```python
from build123d import *

# Parameters (mm, degrees)
F0_W      = 79.8
F0_H      = 79.8
F1_DEPTH  = 15
F2_W      = 74
F2_H      = 74
F3_DEPTH  = 13
F4_W      = 73.8
F4_H      = 73.8
F4_W_2    = 69.8
F4_H_2    = 69.8
F5_DEPTH  = 2
F7_DEPTH  = 2
F8_R      = 2
F9_R      = 4
F10_R     = 0.99999
F12_DEPTH = 79.801
F13_R     = 5
F14_R     = 4
F15_R     = 1


# Not quite as in the source:
# - a fillet or chamfer is up to 0.001 mm smaller than in the source, because OpenCascade refuses the exact size


with BuildPart() as f1:
    # F0 (on Top) → F1 (new body)
    with BuildSketch(Plane.XY):
        Rectangle(F0_W, F0_H)
    extrude(amount=F1_DEPTH)

    # F2 (on face) → F3 (cut)
    with BuildSketch(Plane.XY.offset(15)):
        Rectangle(F2_W, F2_H)
    extrude(amount=-F3_DEPTH, mode=Mode.SUBTRACT)

    # F4 (on face) → F5 (join)
    with BuildSketch(Plane(origin=(0, 0, 0), x_dir=(1, 0, 0), z_dir=(0, 0, -1))):
        Rectangle(F4_W, F4_H)
        Rectangle(F4_W_2, F4_H_2, mode=Mode.SUBTRACT)
    extrude(amount=F5_DEPTH)

    # F6 (on face) → F7 (cut, through all)
    with BuildSketch(Plane(origin=(0, 0, -2), x_dir=(1, 0, 0), z_dir=(0, 0, -1))):
        Polygon((36.9, -21.9), (36.9, 21.9), (21.9, 21.9), (21.9, 36.9), (-21.9, 36.9), (-21.9, 21.9), (-36.9, 21.9), (-36.9, -21.9), (-21.9, -21.9), (-21.9, -36.9), (21.9, -36.9), (21.9, -21.9), align=None)
    extrude(amount=-F7_DEPTH, mode=Mode.SUBTRACT)

    # F8
    f8_edges = [f1.edges().sort_by_distance(p)[0] for p in [
        (-34.9, 34.9, -1),
        (-34.9, -34.9, -1),
        (34.9, -34.9, -1),
        (34.9, 34.9, -1),
    ]]
    fillet(f8_edges, radius=F8_R)

    # F9
    f9_edges = [f1.edges().sort_by_distance(p)[0] for p in [
        (-36.9, 36.9, -1),
        (36.9, 36.9, -1),
        (36.9, -36.9, -1),
        (-36.9, -36.9, -1),
    ]]
    fillet(f9_edges, radius=F9_R)

    # F10 (radius 1 in the source; OpenCascade refuses exactly that, so slightly less here)
    f10_edges = [f1.edges().sort_by_distance(p)[0] for p in [
        (21.9, -35.9, -2),
        (21.9, -35.9, 0),
        (35.9, -21.9, -2),
        (35.9, -21.9, 0),
        (-35.9, -21.9, -2),
        (-35.9, -21.9, 0),
        (-21.9, -35.9, -2),
        (-21.9, -35.9, 0),
        (-35.9, 21.9, -2),
        (-35.9, 21.9, 0),
        (-21.9, 35.9, -2),
        (-21.9, 35.9, 0),
        (21.9, 35.9, -2),
        (21.9, 35.9, 0),
        (35.9, 21.9, -2),
        (35.9, 21.9, 0),
    ]]
    fillet(f10_edges, radius=F10_R)

    # F11 (on face) → F12 (cut, through all)
    with BuildSketch(Plane.XZ.offset(39.9)):
        Polygon((20, 30), (-20, 30), (-12.2222222222, 2), (12.2222222222, 2), align=None)
    extrude(amount=-F12_DEPTH, mode=Mode.SUBTRACT)

    # F13
    f13_edges = [f1.edges().sort_by_distance(p)[0] for p in [
        (-15.833333, 38.45, 15),
        (-15.833333, -38.45, 15),
        (15.833333, -38.45, 15),
        (15.833333, 38.45, 15),
        (-12.222222, 38.45, 2),
        (-12.222222, -38.45, 2),
        (12.222222, -38.45, 2),
        (12.222222, 38.45, 2),
    ]]
    fillet(f13_edges, radius=F13_R)

    # F14
    f14_edges = [f1.edges().sort_by_distance(p)[0] for p in [
        (39.9, -39.9, 7.5),
        (39.9, 39.9, 7.5),
        (-39.9, -39.9, 7.5),
        (-39.9, 39.9, 7.5),
    ]]
    fillet(f14_edges, radius=F14_R)

    # F15
    f15_edges = [f1.edges().sort_by_distance(p)[0] for p in [
        (37, 37, 8.5),
        (-37, 37, 8.5),
        (-37, -37, 8.5),
        (37, -37, 8.5),
    ]]
    fillet(f15_edges, radius=F15_R)


solid = f1.part
```
Work out the finished part from the listing and answer in its coordinate system (mm). A direction names the side the tool comes from. Give positions to 0.01 mm unless a question says otherwise; leave off trailing zeros. Order: outer loops, then holes, each group sorted by start corner. A loop starts at its lowest first (then second) coordinate and runs counter-clockwise, first axis right, second up. Notation, with made-up numbers: (14.25, -3) - (18.25, -3) arc R15 ccw to (18.25, 18) - close; hole circle Ø11 at (74.25, 21). An arc over 180 degrees is marked (long way). One line per item, written item: value. Start each with the question number.
1. Which of the six approach directions +Z, -Z, +X, -X, +Y, -Y give full straight-line access (tool end or side, diameter ignored) to faces 1 (the face through (-37, -1, 9)), 2 (the face through (35.759, 35.697, -1.014)), 3 (the face through (-11.41, -38.43, 2.99)), 4 (the face through (-34.9, -27, -1))?
2. Consider line 1 (Y direction, x = 25, z = 5.75); line 2 (Z direction, x = -35, y = 9). Determine where each line is inside the solid, lowest interval first.
3. Section A-A, the plane y = -7 is taken. Write down the section's boundary in (x, z), then the cut area to 3 significant figures.
4. Section C-C, the plane x = 30.5 is taken. Write down the section's boundary in (y, z), then the cut area to 3 significant figures.
5. Each of these flat-tipped pins is pushed along its axis until it touches: pin 1 Ø5 at (x, y) = (3, -31) entering from +Z; pin 2 Ø0.6 at (x, z) = (24.5, -0.5) entering from +Y; pin 3 Ø2 at (y, z) = (-27.5, -1.5) entering from -X. Where does it stop, or does it pass through?
6. Section B-B, the plane z = 7.75 is taken. Write down the section's boundary in (x, y).
7. For a pull along X with two mould halves and no side action, classify faces 5 (the face through (-35.1, 32.5, -2)), 6 (the face through (11.484, -38.43, 3.047)), 7 (the face through (-38.697, -38.759, 7.605)) as released by +X, released by -X, zero draft, split by the parting line, or undercut.
8. Section D-D, the plane x = -11 is taken. Write down the section's boundary in (y, z).
Filled sheet:
1. face 1: +Z
1. face 2: -Z, +X, +Y
1. face 3: +Z, +Y, -Y
1. face 4: -Z
2. line 1: -39.9 to -37, 37 to 39.9
2. line 2: 0 to 2
3. outline: (-39.9, 0) - (39.9, 0) - (39.9, 15) - (37, 15) - (37, 2) - (-37, 2) - (-37, 15) - (-39.9, 15) - close
3. area: 235 mm²
4. outline: (-39.9, 0) - (-36.9, 0) - (-36.9, -2) - (-34.9, -2) - (-34.9, 0) - (34.9, 0) - (34.9, -2) - (36.9, -2) - (36.9, 0) - (39.9, 0) - (39.9, 15) - (37, 15) - (37, 2) - (-37, 2) - (-37, 15) - (-39.9, 15) - close
4. area: 243 mm²
5. pin 1: z = 2
5. pin 2: y = 36.9
5. pin 3: x = -36.9
6. outline: (-39.9, -35.9) arc R4 ccw to (-35.9, -39.9) - (-13.82, -39.9) - (-13.82, -37) - (-36, -37) arc R1 cw to (-37, -36) - (-37, 36) arc R1 cw to (-36, 37) - (-13.82, 37) - (-13.82, 39.9) - (-35.9, 39.9) arc R4 ccw to (-39.9, 35.9) - close; (13.82, -39.9) - (35.9, -39.9) arc R4 ccw to (39.9, -35.9) - (39.9, 35.9) arc R4 ccw to (35.9, 39.9) - (13.82, 39.9) - (13.82, 37) - (36, 37) arc R1 cw to (37, 36) - (37, -36) arc R1 cw to (36, -37) - (13.82, -37) - close
7. face 5: zero draft
7. face 6: undercut
7. face 7: released by -X
8. outline: (-39.9, 0) - (39.9, 0) - (39.9, 2.72) - (37, 2.72) - (37, 2) - (-37, 2) - (-37, 2.72) - (-39.9, 2.72) - close
